Read the model definition and answer for the solid it produces. Units are mm, in the model's axes. A direction names the side the tool comes from. Round coordinates to 2 decimals unless told otherwise and drop trailing zeros. Write each loop counter-clockwise with the first axis right and the second up, starting at its lowest first coordinate (ties: lowest second). Pieces come first, ordered by that corner, then holes. Notation, with made-up numbers: (60, 23.5) - (118, 23.5) arc R13 cw to (118, 47.5) - close; hole circle Ø3 at (27, -11.5). An arc over 180 degrees is marked (long way). Use one line per item in the form item = value. Start each with the question number.
1) Consider line 1 along Y through (x, z) = (25.4, -23.25); line 2 along Y through (x, z) = (-25, -24); line 3 along X through (y, z) = (107, -6.5). Determine where each line is inside the solid, lowest interval first. Write a range as from..to.
2) The part is cut by section B-B, the plane z = -14. Give the vertices of the cut face in (x, y), plus the area to 3 significant figures.
3) For faces 5 (the face through (-38.1, 63, 0)), 6 (the face through (-27.281, 27.125, -22.181)), 7 (the face through (31.75, 63, 0)), determine the directions among +Z, -Z, +X, -X, +Y, -Y from which every point of the face is accessible in a straight line to the end or side of a thin tool.
4) The part is cut by section A-A, the plane y = 101.6. Give the vertices of the cut face in (x, z).
5) This flat-tipped pin is pushed along its axis until it touches: pin 1 (4 mm diameter, centred on x = 25.4, y = 101.6, fed in from -Z). Where does it stop, or does it pass through?
6) The part is cut by section C-C, the plane x = -25.4. Give the vertices of the cut face in (y, z).
7) For a pull along Y with two mould halves and no side action, classify faces 1 (the face through (-27.281, 103.325, -22.181)), 2 (the face through (-1, 0, 22)), 3 (the face through (-1, 63, -25.4)), 4 (the face through (-1, 127, 22)) as released by +Y, released by -Y, zero draft, split by the parting line, or undercut.
from build123d import *

# Parameters (mm, degrees)
SKETCH1_W                   = 76.2
SKETCH1_H                   = 50.8
SKETCH1_W_2                 = 63.5
SKETCH1_H_2                 = 38.1
BOSS_EXTRUDE1_DEPTH         = 127
F_1_4_20_TAPPED_HOLE1_D     = 5.1054
F_1_4_20_TAPPED_HOLE1_DEPTH = 6.35


with BuildPart() as part:
    # Sketch1 → Boss-Extrude1 (new body)
    with BuildSketch(Plane(origin=(0, 0, 0), x_dir=(1, 0, 0), z_dir=(0, 1, 0))):
        Rectangle(SKETCH1_W, SKETCH1_H)
        Rectangle(SKETCH1_W_2, SKETCH1_H_2, mode=Mode.SUBTRACT)
    extrude(amount=BOSS_EXTRUDE1_DEPTH)

    # 1/4-20 Tapped Hole1
    with Locations(Plane(origin=(0, 0, -25.4), x_dir=(-1, 0, 0), z_dir=(0, 0, -1))):
        with Locations((-25.4, 101.6), (-25.4, 25.4), (25.4, 25.4), (25.4, 101.6)):
            Hole(F_1_4_20_TAPPED_HOLE1_D / 2, depth=F_1_4_20_TAPPED_HOLE1_DEPTH)


solid = part.part
Geometry results:
q1.line_1 = 0..22.85, 27.95..99.05, 104.15..127
q1.line_2 = 0..22.88, 27.92..99.08, 104.12..127
q1.line_3 = -38.1..-31.75, 31.75..38.1
q2.outline = (-38.1, 0) - (-31.75, 0) - (-31.75, 127) - (-38.1, 127) - close; (31.75, 0) - (38.1, 0) - (38.1, 127) - (31.75, 127) - close
q2.area = 1,610 mm2
q3.face_5 = +Z, -Z, -X, +Y, -Y
q3.face_6 = -Z
q3.face_7 = +Y, -Y
q4.outline = (-38.1, -25.4) - (-27.95, -25.4) - (-27.95, -19.05) - (-31.75, -19.05) - (-31.75, 19.05) - (31.75, 19.05) - (31.75, -19.05) - (27.95, -19.05) - (27.95, -25.4) - (38.1, -25.4) - (38.1, 25.4) - (-38.1, 25.4) - close; (-22.85, -25.4) - (22.85, -25.4) - (22.85, -19.05) - (-22.85, -19.05) - close
q5.pin_1 = 19.05
q6.outline = (0, -25.4) - (22.85, -25.4) - (22.85, -19.05) - (0, -19.05) - close; (0, 19.05) - (127, 19.05) - (127, 25.4) - (0, 25.4) - close; (27.95, -25.4) - (99.05, -25.4) - (99.05, -19.05) - (27.95, -19.05) - close; (104.15, -25.4) - (127, -25.4) - (127, -19.05) - (104.15, -19.05) - close
q7.face_1 = undercut
q7.face_2 = released by -Y
q7.face_3 = zero draft
q7.face_4 = released by +Y
